Input: dimensioned drawing with shaded views. Units: mm. Origin: part minimum x, y, z. A direction names the side the tool comes from. Round coordinates to 2 decimals unless told otherwise and drop trailing zeros. Loops run counter-clockwise (first coordinate to the right, second up) from the corner with the lowest first, then second, coordinate; pieces in that order, holes last. Notation, with made-up numbers: M 45.25,47.25 L 60.25,47.25 A28 cw 60.25,79.25 Z; hole C 40.25,-22.5 d6. An arc over 180 degrees is marked long. One line per item, written item: value.
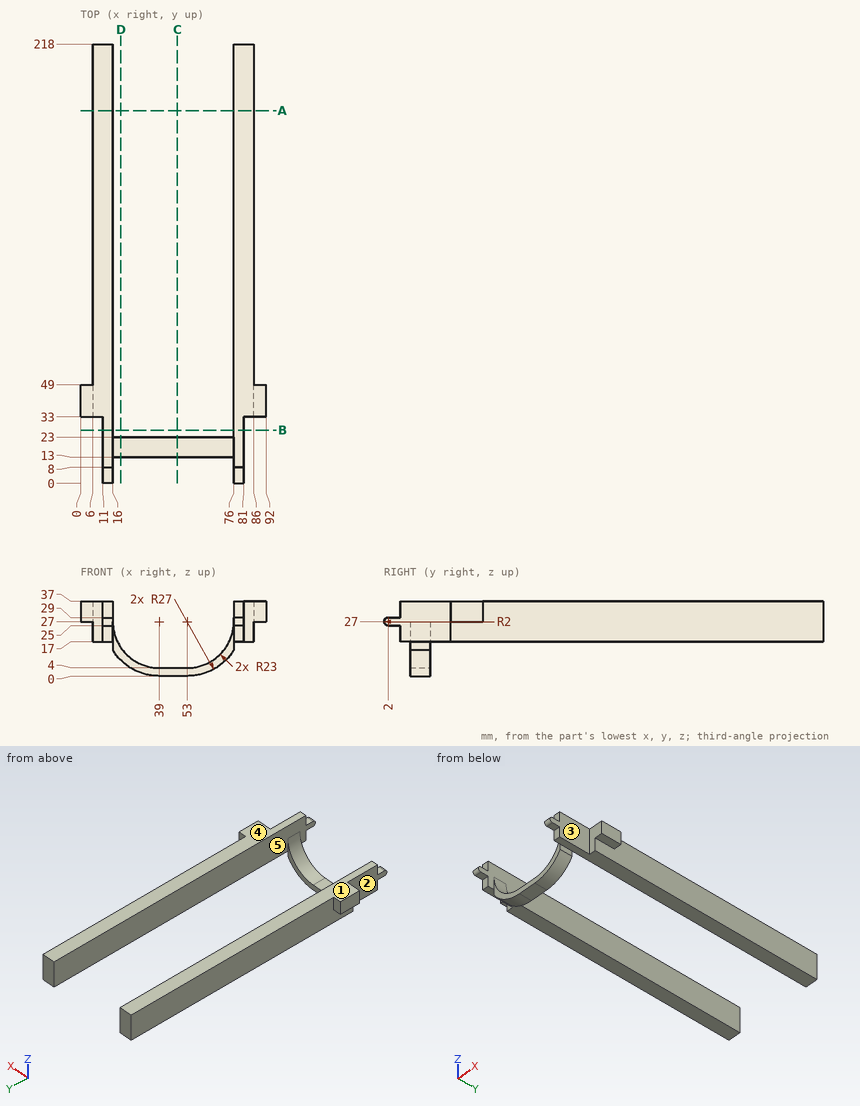
1. Section query A-A (y = 185). Return the cut outline in (x, z).
Report:
outline: M 6,17 L 16,17 L 16,37 L 6,37 Z; M 76,17 L 86,17 L 86,37 L 76,37 Z
2. Section query D-D (x = 20). Return the cut outline in (y, z).
Report:
outline: M 13,7.82 L 23,7.82 L 23,14.04 L 13,14.04 Z
3. Pin query (flat end, axial travel): pin 1 (9 mm diameter, centred on x = 87.5, z = 24, fed in from -Y); pin 2 (6 mm diameter, centred on y = 115, z = 24, fed in from -X); pin 3 (3 mm diameter, centred on x = 48, y = 17.5, fed in from +Z). Return the tip coordinate at first contact, or that it passes through.
Report:
pin 1: stops at y = 33
pin 2: stops at x = 6
pin 3: stops at z = 4
4. Ray query, line 1 (X direction, y = 170.5, z = 28); line 2 (Y direction, x = 10.5, z = 34.5); line 3 (Z direction, x = 88.5, y = 43). Return the intervals inside material, ascending. Write a range as [from, to].
Report:
line 1: x = [6, 16], [76, 86]
line 2: y = [33, 218]
line 3: z = [27, 37]
5. Section query C-C (x = 48). Return the cut outline in (y, z), and give its area (3 significant figures).
Report:
outline: M 13,0 L 23,0 L 23,4 L 13,4 Z
area: 40.0 mm2
6. Reachability of the marked faces 1 and 2 from +Z, -Z, +X, -X, +Y, -Y: full face, straight path, thin tool, end or side. Return the list, or none.
Report:
face 1: +Z, +X, -X, +Y, -Y
face 2: +Z, -Z, -X, -Y
7. Section query B-B (y = 26.5). Return the cut outline in (x, z), and give its area (3 significant figures).
Report:
outline: M 11,17 L 16,17 L 16,37 L 11,37 Z; M 76,17 L 81,17 L 81,37 L 76,37 Z
area: 200 mm2
8. Pull-direction query (X, two-part tool) for the marked faces 3, 4 and 5; classes: released by +X, released by -X, zero draft, split by the parting line, or undercut.
Report:
face 3: released by +X
face 4: zero draft
face 5: undercut
